from build123d import *

# Parameters (mm, degrees)
SKETCH1_W               = 65
SKETCH1_H               = 50
BOSS_EXTRUDE1_DEPTH     = 10
SKETCH2_W               = 15
SKETCH2_H               = 50
BOSS_EXTRUDE2_DEPTH     = 70
CUT_EXTRUDE1_DEPTH      = 107.77078252
CUT_EXTRUDE1_DEPTH_BACK = 107.77078252
SKETCH3_R               = 10
BOSS_EXTRUDE7_REACH     = 108.771
FILLET1_R               = 1
SKETCH6_W               = 25
SKETCH6_H               = 50
BOSS_EXTRUDE8_DEPTH     = 150
SKETCH7_R               = 12.5
CUT_EXTRUDE2_DEPTH      = 150
SKETCH8_W               = 15
SKETCH8_H               = 50
CUT_EXTRUDE3_DEPTH      = 150
SKETCH11_W              = 25
SKETCH11_H              = 50
BOSS_EXTRUDE9_DEPTH     = 150
SKETCH12_R              = 15
CUT_EXTRUDE4_DEPTH      = 150
BOSS_EXTRUDE10_DEPTH    = 15


with BuildPart() as part:
    # Sketch1 → Boss-Extrude1 (new body)
    with BuildSketch(Plane(origin=(0, 0, 0), x_dir=(1, 0, 0), z_dir=(0, 1, 0))):
        with Locations((-32.5, 25)):
            Rectangle(SKETCH1_W, SKETCH1_H)
    extrude(amount=BOSS_EXTRUDE1_DEPTH)

    # Sketch2 → Boss-Extrude2 (add)
    with BuildSketch(Plane(origin=(0, 10, 0), x_dir=(1, 0, 0), z_dir=(0, 1, 0))):
        with Locations((-57.5, 25)):
            Rectangle(SKETCH2_W, SKETCH2_H)
        with Locations((-7.5, 25)):
            Rectangle(SKETCH2_W, SKETCH2_H)
    extrude(amount=BOSS_EXTRUDE2_DEPTH)

    # Sketch3 → Cut-Extrude1 (cut, two sides: drawn at the far end of the back side and taken through both)
    with BuildSketch(Plane(origin=(-50, 0, 0), x_dir=(0, 0, -1), z_dir=(1, 0, 0)).offset(-CUT_EXTRUDE1_DEPTH_BACK)):
        with Locations((25, 65)):
            Circle(SKETCH3_R)
    extrude(amount=CUT_EXTRUDE1_DEPTH + CUT_EXTRUDE1_DEPTH_BACK, mode=Mode.SUBTRACT)

    # Sketch5 → Boss-Extrude7 (add, up to next)
    with BuildSketch(Plane(origin=(-50, 0, 0), x_dir=(0, 0, -1), z_dir=(1, 0, 0)), mode=Mode.PRIVATE) as boss_extrude7_sk1:
        with BuildLine():
            Line((50, 10), (50, 35))
            ThreePointArc((50, 35), (42.67766953, 17.32233047), (25, 10))
            Line((25, 10), (50, 10))
        make_face()
    boss_extrude7_tool1 = extrude(boss_extrude7_sk1.sketch, amount=BOSS_EXTRUDE7_REACH, mode=Mode.PRIVATE) - part.part
    # Sketch5 → Boss-Extrude7 (add, up to next)
    with BuildSketch(Plane(origin=(-50, 0, 0), x_dir=(0, 0, -1), z_dir=(1, 0, 0)), mode=Mode.PRIVATE) as boss_extrude7_sk2:
        with BuildLine():
            ThreePointArc((25, 10), (7.32233047, 17.32233047), (0, 35))
            Line((0, 35), (0, 10))
            Line((0, 10), (25, 10))
        make_face()
    boss_extrude7_tool2 = extrude(boss_extrude7_sk2.sketch, amount=BOSS_EXTRUDE7_REACH, mode=Mode.PRIVATE) - part.part
    add(boss_extrude7_tool1.solids().sort_by_distance((-50, 15.584198, -44.415802))[0])
    add(boss_extrude7_tool2.solids().sort_by_distance((-50, 15.584198, -5.584198))[0])

    # Fillet1
    fillet1_edges = [part.edges().sort_by_distance(p)[0] for p in [
        (-32.5, 35, -50),
        (-32.5, 35, 0),
    ]]
    fillet(fillet1_edges, radius=FILLET1_R)

    # Sketch6 → Boss-Extrude8 (add)
    with BuildSketch(Plane.XZ):
        with Locations((-52.5, -25)):
            Rectangle(SKETCH6_W, SKETCH6_H)
    extrude(amount=BOSS_EXTRUDE8_DEPTH)

    # Sketch7 → Cut-Extrude2 (cut)
    with BuildSketch(Plane(origin=(-40, 0, 0), x_dir=(0, 0, -1), z_dir=(1, 0, 0))):
        with Locations((25, -126.825479142)):
            Circle(SKETCH7_R)
    extrude(amount=-CUT_EXTRUDE2_DEPTH, mode=Mode.SUBTRACT)

    # Sketch8 → Cut-Extrude3 (cut)
    with BuildSketch(Plane.XZ):
        with Locations((-32.5, -25)):
            Rectangle(SKETCH8_W, SKETCH8_H)
    extrude(amount=-CUT_EXTRUDE3_DEPTH, mode=Mode.SUBTRACT)


with BuildPart() as cut_extrude3_piece_1:
    # of the separate pieces the step leaves, piece 1, a body of its own (cut_extrude3_pieces)
    add(part.part.solids().sort_by_distance((-50, 25, 0))[0])



with BuildPart() as cut_extrude3_piece_2:
    # of the separate pieces the step leaves, piece 2, a body of its own (cut_extrude3_pieces)
    add(part.part.solids().sort_by_distance((-25, 25, 0))[0])

    # Sketch11 → Boss-Extrude9 (add)
    with BuildSketch(Plane.XZ):
        with Locations((-12.5, -25)):
            Rectangle(SKETCH11_W, SKETCH11_H)
    extrude(amount=BOSS_EXTRUDE9_DEPTH)

    # Sketch12 → Cut-Extrude4 (cut)
    with BuildSketch(Plane.ZY.offset(25)):
        with Locations((-25, -126.825479142)):
            Circle(SKETCH12_R)
    extrude(amount=-CUT_EXTRUDE4_DEPTH, mode=Mode.SUBTRACT)


with BuildPart() as cut_extrude3_piece_1_1:
    add(cut_extrude3_piece_1.part)

    add(cut_extrude3_piece_2.part)  # Boss-Extrude10 merges Cut-Extrude3 piece 2
    # Sketch14 → Boss-Extrude10 (add)
    with BuildSketch(Plane.ZY.offset(25)):
        with BuildLine():
            Line((-5, -126.825479142), (0, -126.825479142))
            Line((0, -126.825479142), (0, -150))
            Line((0, -150), (-50, -150))
            Line((-50, -150), (-50, -126.825479142))
            Line((-50, -126.825479142), (-45, -126.825479142))
            ThreePointArc((-45, -126.825479142), (-25, -146.825479142), (-5, -126.825479142))
        make_face()
    extrude(amount=BOSS_EXTRUDE10_DEPTH)


solid = cut_extrude3_piece_1_1.part
CAD build for the part. Positions are in the model's coordinates, mm. A direction names the side the tool comes from. Coordinates: 2 decimals unless noted, no trailing zeros. Write each loop counter-clockwise with the first axis right and the second up, starting at its lowest first coordinate (ties: lowest second). Pieces come first, ordered by that corner, then holes. Notation, with made-up numbers: M 9,32 L 67,32 A15 cw 67,46 Z; hole C 74,55 d8. An arc over 180 degrees is marked long. Answer as a JSON object with one key per item and string values. Group by question number.
1) Saw through at B-B (z = -28.5). Write the cut outline in (x, y).
2) Tool access for faces 1 (the face through (-12.68, -141.47, -28.25)), 2 (the face through (-32, -126.825, -3)), 3 (the face through (-15, 45, -25)): list every direction of +Z, -Z, +X, -X, +Y, -Y with a clear straight run to the whole face (end or side of a thin tool).
3) Saw through at C-C (y = -135). Write the cut outline in (x, z).
4) Pin check, flat tips, straight feed: pin 1 Ø2.5 at (x, z) = (-29.5, -3.5) entering from +Y; pin 2 Ø16 at (y, z) = (65, -25) entering from +X; pin 3 Ø4 at (x, z) = (-41.5, -10) entering from +Y; pin 4 Ø4 at (x, z) = (-35.5, -30.5) entering from +Y. Stop position of each tip, or through.
5) Wall check: line 1 (Y direction, x = -54, z = -25); line 2 (Z direction, x = -8, y = 65); line 3 (X direction, y = 10, z = -40). Give the ranges that are in metal, low to high. Write a range as from..to.
6) Saw through at D-D (x = -37.5). Write the cut outline in (y, z).
7) Saw through at A-A (y = 65). Write the cut outline in (x, z).
8) Mould opens along X. For faces 4 (the face through (-32, -126.825, -48)), 5 (the face through (-65, -33, -25)), 6 (the face through (-8, 80, -25)) say: +X half, -X half, draft (parallel to the pull), parting line (faces both ways), or undercut.
Values follow:
{
 "1": {"outline": "M -65,-150 L 0,-150 L 0,-141.41 L -25,-141.41 L -25,-146.52 L -40,-146.52 L -40,-138.83 L -65,-138.83 Z; M -65,-114.83 L -40,-114.83 L -40,10.25 L -50,10.25 L -50,55.63 L -65,55.63 Z; M -65,74.37 L -50,74.37 L -50,80 L -65,80 Z; M -25,-112.24 L 0,-112.24 L 0,55.63 L -15,55.63 L -15,10.25 L -25,10.25 Z; M -15,74.37 L 0,74.37 L 0,80 L -15,80 Z"},
 "2": {"face 1": "+X", "face 2": "+Z, -Z, +Y", "face 3": "+Y"},
 "3": {"outline": "M -65,-50 L 0,-50 L 0,-37.58 L -25,-37.58 L -25,-43.25 L -40,-43.25 L -40,-34.46 L -65,-34.46 Z; M -65,-15.54 L -40,-15.54 L -40,-6.75 L -25,-6.75 L -25,-12.42 L 0,-12.42 L 0,0 L -65,0 Z"},
 "4": {"pin 1": "stops at y = -126.83", "pin 2": "passes through", "pin 3": "stops at y = 16.67", "pin 4": "stops at y = -145.37"},
 "5": {"line 1": "y = -150..-139.33, -114.33..55, 75..80", "line 2": "z = -50..-35, -15..0", "line 3": "x = -65..-40, -25..0"},
 "6": {"outline": "M -150,-50 L -126.83,-50 L -126.83,-45 A20 cw -126.83,-5 L -126.83,0 L -150,0 Z"},
 "7": {"outline": "M -65,-50 L -50,-50 L -50,-35 L -65,-35 Z; M -65,-15 L -50,-15 L -50,0 L -65,0 Z; M -15,-50 L 0,-50 L 0,-35 L -15,-35 Z; M -15,-15 L 0,-15 L 0,0 L -15,0 Z"},
 "8": {"face 4": "undercut", "face 5": "-X half", "face 6": "draft"}
}
